Verification items for the finished model (mm, model axes). A direction names the side the tool comes from. Coordinates: 2 decimals unless noted, no trailing zeros. Order: outer loops, then holes, each group sorted by start corner. A loop starts at its lowest first (then second) coordinate and runs counter-clockwise, first axis right, second up. Notation, with made-up numbers: (84.5, 25.25) -> (140.5, 25.25) arc R6 ccw to (140.5, 33.25) -> close; hole circle Ø6 at (-16, 1). An arc over 180 degrees is marked (long way). Write item = value, one per line. Start each with the question number.
from build123d import *

# Parameters (mm, degrees)
F1_DEPTH = 25.3
F2_DEPTH = 25


with BuildPart() as f1:
    # F0 (on Front) → F1 (new body)
    with BuildSketch(Plane.XZ):
        with BuildLine():
            ThreePointArc((-47.4482923746, 31.4433462918), (-74.5009016246, 4.3907370418), (-47.4482923746, -22.6618722081))
            Line((-47.4482923746, -22.6618722081), (0, -22.6618722081))
            Line((0, -22.6618722081), (0, 31.4433462918))
            Line((0, 31.4433462918), (-47.4482923746, 31.4433462918))
        make_face()
    extrude(amount=F1_DEPTH)

    # F2 (add): faces of the model
    f2_faces = [f1.faces().sort_by_distance(p)[0] for p in [
        (-23.7241461873, -12.65, -22.6618722081),
        (-23.7241461873, -12.65, 31.4433462918),
    ]]
    extrude(f2_faces, amount=F2_DEPTH, dir=(0, 0, -1))


solid = f1.part
Item 1: Section check B-B (z = -28). Record the boundary of the cut face in (x, y).
Item 2: Tool access check on faces 1 (the flat face through (-29, -25.3, -8)), 2 (the flat face through (-47.448, -12, -35)). Record the directions out of +Z, -Z, +X, -X, +Y, -Y that give a thin tool (end or side, any length) a straight path to the whole face; none if there is none.
Item 3: Section check C-C (x = -65.5). Record the boundary of the cut face in (y, z).
Item 4: Section check A-A (y = -19). Record the boundary of the cut face in (x, z), then the cut area to 3 significant figures.
Item 5: Thickness scan on line 1 (X direction, y = -21.5, z = -35.5); line 2 (X direction, y = -3.75, z = 17); line 3 (Z direction, x = -63.5, y = -13.5). Record the ranges inside material, lowest first.
Item 6: Gauge pin test, flat ends, axial feed: P1, Ø6, axis at y = -3, z = -10, coming from the -X side; P2, Ø6, axis at y = -11.5, z = -33, coming from the -X side; P3, Ø1.5, axis at y = -15, z = -7.5, coming from the -X side. Record the tip position at first contact, or that the pin passes through.
Filled sheet:
q1.outline = (-47.45, -25.3) -> (0, -25.3) -> (0, 0) -> (-47.45, 0) -> close
q2.face_1 = +Z, -Z, +X, -X, -Y
q2.face_2 = -Z, -X, +Y, -Y
q3.outline = (-25.3, -15.76) -> (0, -15.76) -> (0, 24.54) -> (-25.3, 24.54) -> close
q4.outline = (-47.45, -47.66) -> (0, -47.66) -> (0, 31.44) -> (-47.45, 31.44) arc R27.05 ccw to (-47.45, -22.66) -> close
q4.area = 4,900 mm^2
q5.line_1 = -47.45 to 0
q5.line_2 = -71.38 to 0
q5.line_3 = -17.39 to 26.17
q6.P1 = -71.99
q6.P2 = -47.45
q6.P3 = -72.1
